Geometry check sheet. Reference: the model listing, model coordinates, mm. A direction names the side the tool comes from. Coordinates: 2 decimals unless noted, no trailing zeros. Loops run counter-clockwise (first coordinate to the right, second up) from the corner with the lowest first, then second, coordinate; pieces in that order, holes last.
from build123d import *

# Parameters (mm, degrees)
F0_W     = 77.067762
F0_H     = 46.12676
F0_R     = 5.950275
F0_R_2   = 5.930231
F0_R_3   = 5.905875
F1_DEPTH = 22.86
F2_DEPTH = 27.94
F3_DEPTH = 27.94
F4_DEPTH = 10


with BuildPart() as f1:
    # F0 (on Top) → F1 (new body)
    with BuildSketch(Plane.XY):
        Rectangle(F0_W, F0_H)
        with Locations((-24.487047, -10.914768)):
            Circle(F0_R, mode=Mode.SUBTRACT)
        with Locations((0, -10.914768)):
            Circle(F0_R_2, mode=Mode.SUBTRACT)
        with Locations((25.469103, -10.914768)):
            Circle(F0_R_3, mode=Mode.SUBTRACT)
        with Locations((-24.487047, 10.914768)):
            Circle(F0_R, mode=Mode.SUBTRACT)
        with Locations((0, 10.914768)):
            Circle(F0_R_2, mode=Mode.SUBTRACT)
        with Locations((25.469103, 10.914768)):
            Circle(F0_R_3, mode=Mode.SUBTRACT)
    extrude(amount=F1_DEPTH)

    # F0 (on Top) → F2 (join)
    with BuildSketch(Plane.XY):
        with Locations((-24.487047, 10.914768)):
            Circle(F0_R)
        with Locations((0, 10.914768)):
            Circle(F0_R_2)
        with Locations((25.469103, 10.914768)):
            Circle(F0_R_3)
        with Locations((25.469103, -10.914768)):
            Circle(F0_R_3)
        with Locations((0, -10.914768)):
            Circle(F0_R_2)
        with Locations((-24.487047, -10.914768)):
            Circle(F0_R)
    extrude(amount=F2_DEPTH)

    # F0 (on Top) → F3 (join, through all)
    with BuildSketch(Plane.XY):
        with Locations((-24.487047, 10.914768)):
            Circle(F0_R)
        with Locations((-24.487047, -10.914768)):
            Circle(F0_R)
        with Locations((0, -10.914768)):
            Circle(F0_R_2)
        with Locations((0, 10.914768)):
            Circle(F0_R_2)
        with Locations((25.469103, 10.914768)):
            Circle(F0_R_3)
        with Locations((25.469103, -10.914768)):
            Circle(F0_R_3)
    extrude(amount=F3_DEPTH)

    # F0 (on Top) → F4 (cut)
    with BuildSketch(Plane.XY):
        with Locations((-24.487047, -10.914768)):
            Circle(F0_R)
        with Locations((0, -10.914768)):
            Circle(F0_R_2)
        with Locations((25.469103, -10.914768)):
            Circle(F0_R_3)
        with Locations((25.469103, 10.914768)):
            Circle(F0_R_3)
        with Locations((0, 10.914768)):
            Circle(F0_R_2)
        with Locations((-24.487047, 10.914768)):
            Circle(F0_R)
    extrude(amount=F4_DEPTH, mode=Mode.SUBTRACT)


solid = f1.part
1) Section check D-D on z = 6.75. Record the cut outline in (x, y).
Data:
outline: (-38.53, -23.06) - (38.53, -23.06) - (38.53, 23.06) - (-38.53, 23.06) - close; hole circle Ø11.9 at (-24.49, -10.91); hole circle Ø11.9 at (-24.49, 10.91); hole circle Ø11.86 at (0, -10.91); hole circle Ø11.86 at (0, 10.91); hole circle Ø11.81 at (25.47, -10.91); hole circle Ø11.81 at (25.47, 10.91)
2) Material ranges on probe 1 along Y at (x, z) = (0, 6.25) (3 decimals); probe 2 along Y at (x, z) = (-27, 2.25); probe 3 along X at (y, z) = (9, 2.25), recorded low to high.
Data:
probe 1: y = -23.063 to -16.845, -4.985 to 4.985, 16.845 to 23.063
probe 2: y = -23.06 to -16.31, -5.52 to 5.52, 16.31 to 23.06
probe 3: x = -38.53 to -30.12, -18.85 to -5.61, 5.61 to 19.88, 31.06 to 38.53
3) Depth check by flat-ended pin: pin 1 (10.5 mm diameter, centred on x = 0, y = 10.91, fed in from -Z); pin 2 (6 mm diameter, centred on x = -13.5, y = 10, fed in from +Z); pin 3 (14 mm diameter, centred on x = -7.5, y = 5, fed in from +Z). Enter the tip coordinate at first touch or a pass-through.
Data:
pin 1: stops at z = 10
pin 2: stops at z = 22.86
pin 3: stops at z = 27.94
4) Section check C-C on y = 3. Record the cut outline in (x, z).
Data:
outline: (-38.53, 0) - (38.53, 0) - (38.53, 22.86) - (-38.53, 22.86) - close
5) Mould release check, pull along Y, two halves, no side actions. Record for faces 1 (the flat face through (0, -11, 27.94)), 2 (the cylindrical face through (-1.286, 5.126, 25.364)), 3 (the flat face through (-1, 23.063, 11)): +Y half, -Y half, draft (parallel to the pull), parting line (faces both ways), or undercut.
Data:
face 1: draft
face 2: undercut
face 3: +Y half
6) Section check B-B on x = 0. Record the cut outline in (y, z) (3 decimals).
Data:
outline: (-23.063, 0) - (-16.845, 0) - (-16.845, 10) - (-4.985, 10) - (-4.985, 0) - (4.985, 0) - (4.985, 10) - (16.845, 10) - (16.845, 0) - (23.063, 0) - (23.063, 22.86) - (16.845, 22.86) - (16.845, 27.94) - (4.985, 27.94) - (4.985, 22.86) - (-4.985, 22.86) - (-4.985, 27.94) - (-16.845, 27.94) - (-16.845, 22.86) - (-23.063, 22.86) - close
7) Access from +Z, -Z, +X, -X, +Y, -Y to the whole of each face (thin tool, end or side, straight path). Record for faces 4 (the cylindrical face through (-0.772, -5.035, 25.364)), 5 (the flat face through (25, -11, 27.94)), 6 (the cylindrical face through (24.19, -16.68, 4.93)).
Data:
face 4: +Z
face 5: +Z, +X, -X, +Y, -Y
face 6: -Z
8) Section check A-A on z = 25.25. Record the cut outline in (x, y), and give its area (3 significant figures).
Data:
outline: circle Ø11.9 at (-24.49, -10.91); circle Ø11.9 at (-24.49, 10.91); circle Ø11.86 at (0, -10.91); circle Ø11.86 at (0, 10.91); circle Ø11.81 at (25.47, -10.91); circle Ø11.81 at (25.47, 10.91)
area: 663 mm2
